Can you work these out from the model? Positions are in its coordinate system, mm. Round coordinates to 2 decimals unless told otherwise and drop trailing zeros. Write each loop counter-clockwise with the first axis right and the second up, starting at its lowest first coordinate (ties: lowest second). Pieces come first, ordered by that corner, then holes. Notation, with made-up numbers: M 28.25,-22 L 55.25,-22 A20 ccw 55.25,-6 Z; hole C -10,-18.5 d9. An arc over 180 degrees is marked long. Answer in a Markdown table with one row per item. Add a question column.
(1) If I drill on probe 1 along Y at (x, z) = (4.75, 0) (3 decimals); probe 2 along Y at (x, z) = (-4.5, -0.5); probe 3 along X at (y, z) = (382, 0.5), over which ranges is the centre line in solid material (lowest first)?
(2) I'm going to push flat-ended pins straight in: pin 1 (3 mm diameter, centred on y = 93, z = -4, fed in from +X); pin 2 (1.5 mm diameter, centred on x = -1.5, y = 247.5, fed in from -Z); pin 3 (5 mm diameter, centred on y = 407.5, z = 3, fed in from -X). Where does each tip first touch, or does it pass through?
(3) Suppose I cut it at B-B, the plane y = 331. Write out the boundary of the cut face in (x, z), then the cut area to 3 significant figures.
(4) Suppose I cut it at A-A, the plane z = 0. Write out the boundary of the cut face in (x, y) (3 decimals), then the cut area to 3 significant figures.
from build123d import *

# Parameters (mm, degrees)
SKETCH1_R               = 6.35
BOSS_EXTRUDE1_DEPTH     = 457.2
SKETCH2_R               = 3.175
CUT_EXTRUDE1_DEPTH      = 7.35
CUT_EXTRUDE1_DEPTH_BACK = 7.35


with BuildPart() as part:
    # Sketch1 → Boss-Extrude1 (new body)
    with BuildSketch(Plane(origin=(0, 0, 0), x_dir=(1, 0, 0), z_dir=(0, 1, 0))):
        with Locations(Location((0, 0, 0), (0, 0, 270))):  # turned: the seam where the file's is
            Circle(SKETCH1_R)
    extrude(amount=BOSS_EXTRUDE1_DEPTH)

    # Sketch2 → Cut-Extrude1 (cut, two sides)
    with BuildSketch(Plane(origin=(0, 0, 0), x_dir=(0, 0, -1), z_dir=(1, 0, 0))) as cut_extrude1_sk:
        with Locations((0, 25.4)):
            Circle(SKETCH2_R)
        with Locations((0, 127)):
            Circle(SKETCH2_R)
    extrude(amount=CUT_EXTRUDE1_DEPTH, mode=Mode.SUBTRACT)
    extrude(cut_extrude1_sk.sketch, amount=-CUT_EXTRUDE1_DEPTH_BACK, mode=Mode.SUBTRACT)


solid = part.part
Calculated:
| question | item | result |
|---|---|---|
| 1 | probe 1 | 0 to 22.225, 28.575 to 123.825, 130.175 to 457.2 |
| 1 | probe 2 | 0 to 22.26, 28.54 to 123.86, 130.14 to 457.2 |
| 1 | probe 3 | -6.33 to 6.33 |
| 2 | pin 1 | x = 5.84 |
| 2 | pin 2 | z = -6.31 |
| 2 | pin 3 | x = -6.33 |
| 3 | outline | C 0,0 d12.7 |
| 3 | area | 127 mm² |
| 4 | outline | M -6.35,0 L 6.35,0 L 6.35,22.225 L -6.35,22.225 Z; M -6.35,28.575 L 6.35,28.575 L 6.35,123.825 L -6.35,123.825 Z; M -6.35,130.175 L 6.35,130.175 L 6.35,457.2 L -6.35,457.2 Z |
| 4 | area | 5,650 mm² |
